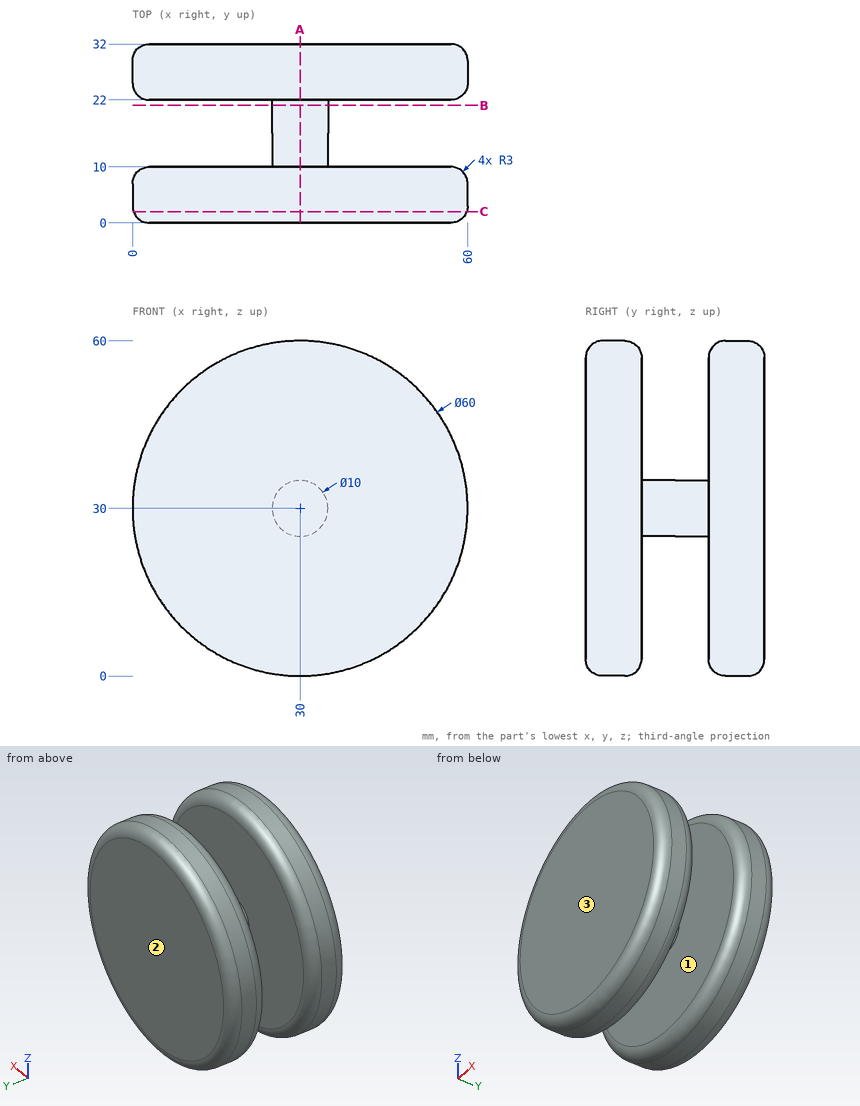
Answer from the drawing. Dimensions are ordinates in mm from the lowest x, y and z of the part. Round coordinates to 2 decimals unless told otherwise and drop trailing zeros. Write each loop counter-clockwise with the first axis right and the second up, starting at its lowest first coordinate (ties: lowest second). Pieces come first, ordered by that corner, then holes.
1. Given pin 1 Ø12 at (y, z) = (18.5, 27) entering from +X; pin 2 Ø4 at (y, z) = (24, 8.5) entering from +X; pin 3 Ø1.5 at (x, y) = (7, 4.5) entering from +Z, each flat-ended and moving along its own axis, determine where each tip first touches the part or whether it passes through.
2. The part is cut by section C-C, the plane y = 2. Determine the outline of the cut face in (x, z).
3. The part is cut by section A-A, the plane x = 30. Determine the outline of the cut face in (y, z).
4. Determine the mould class of the marked faces 1, 2 and 3 for opening direction Y: pulls with the +Y half, pulls with the -Y half, needs draft (parallel to the pull), parting line crosses it, or undercut.
5. Straight lines are drawn through the part: L1, parallel to Y at x = 21, z = 27.5; L2, parallel to Y at x = 10.5, z = 50.5; L3, parallel to Z at x = 24.5, y = 31. For each, find the intervals that lie inside material, in ascending order.
6. The part is cut by section B-B, the plane y = 21. Determine the outline of the cut face in (x, z).
Values:
1. pin 1: stops at x = 59.88
1. pin 2: stops at x = 52.69
1. pin 3: stops at z = 50.12
2. outline: circle Ø59.66 at (30, 30)
3. outline: (0, 3) arc R3 ccw to (3, 0) - (7, 0) arc R3 ccw to (10, 3) - (10, 25) - (22, 25) - (22, 3) arc R3 ccw to (25, 0) - (29, 0) arc R3 ccw to (32, 3) - (32, 57) arc R3 ccw to (29, 60) - (25, 60) arc R3 ccw to (22, 57) - (22, 35) - (10, 35) - (10, 57) arc R3 ccw to (7, 60) - (3, 60) arc R3 ccw to (0, 57) - close
4. face 1: undercut
4. face 2: pulls with the +Y half
4. face 3: pulls with the -Y half
5. L1: y = 0 to 10, 22 to 32
5. L2: y = 0.29 to 9.71, 22.29 to 31.71
5. L3: z = 1.29 to 58.71
6. outline: circle Ø10 at (30, 30)
